Job drawing, mm, ordinate dimensions from the low corner. One solid piece. A direction names the side the tool comes from. Give positions to 0.01 mm unless a question says otherwise; leave off trailing zeros. Write each loop counter-clockwise with the first axis right and the second up, starting at its lowest first coordinate (ties: lowest second). Pieces come first, ordered by that corner, then holes. Notation, with made-up numbers: M 5,46 L 54,46 A16 ccw 54,69 Z; hole C 2,80.25 d8. An arc over 180 degrees is marked long. Answer as CSV lines item,"result". Start each with the question number.
Item 1: Wall check: L1, parallel to Y at x = 14, z = 10.6; L2, parallel to X at y = 15, z = 8.5 (1 decimal); L3, parallel to Z at x = 17.5, y = 22. Give the ranges that are in metal, low to high. Write a range as from..to.
Item 2: Band-saw the part on A-A, the plane y = 14. Count the separate pieces of the cut face and the enclosed holes in it.
Item 3: Band-saw the part on D-D, the plane x = 9.5. List the corners of the cut face in (y, z).
Item 4: Pin check, flat tips, straight feed: pin 1 (10 mm diameter, centred on y = 7.5, z = 9.5, fed in from +X); pin 2 (1.5 mm diameter, centred on y = 9.5, z = 16.5, fed in from +X); pin 3 (5 mm diameter, centred on x = 25, y = 14, fed in from +Z); pin 4 (1.8 mm diameter, centred on x = 14, y = 3, fed in from +Z). Stop position of each tip, or through.
Item 5: Band-saw the part on B-B, the plane x = 3. List the corners of the cut face in (y, z).
Item 6: 3-axis set-ups, long thin cutter, end or side, ignore diameter. For the marked faces 1, 2 and 3: which of +Z, -Z, +X, -X, +Y, -Y reach the whole face in a straight line?
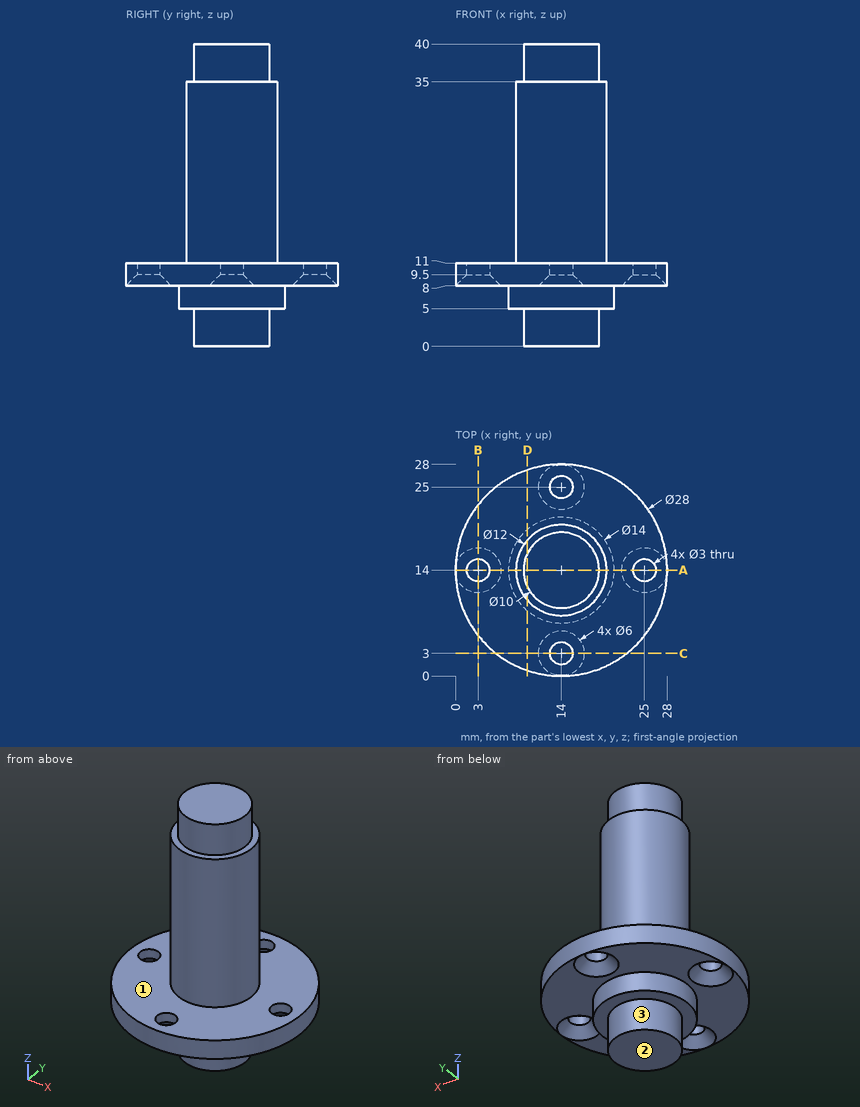
Output:
1,L1,"0..1.5, 4.5..23.5, 26.5..28"
1,L2,"0..0.7, 5.3..22.7, 27.3..28"
1,L3,"8..11"
2,separate pieces,"3"
2,enclosed holes,"0"
3,outline,"M 0.74,8 L 8.64,8 L 8.64,5 L 11.82,5 L 11.82,0 L 16.18,0 L 16.18,5 L 19.36,5 L 19.36,8 L 27.26,8 L 27.26,11 L 17.97,11 L 17.97,35 L 16.18,35 L 16.18,40 L 11.82,40 L 11.82,35 L 10.03,35 L 10.03,11 L 0.74,11 Z"
4,pin 1,"x = 27.92"
4,pin 2,"x = 18.68"
4,pin 3,"z = 11"
4,pin 4,"through"
5,outline,"M 5.34,8 L 11,8 L 12.5,9.5 L 12.5,11 L 5.34,11 Z; M 15.5,9.5 L 17,8 L 22.66,8 L 22.66,11 L 15.5,11 Z"
6,face 1,"+Z"
6,face 2,"-Z, +X, -X, +Y, -Y"
6,face 3,"-Z"
